from build123d import *

# Parameters (mm, degrees)
BOSS_EXTRUDE1_DEPTH      = 14.5
BOSS_EXTRUDE1_DEPTH_BACK = 14.5
SKETCH2_R                = 1.205
BOSS_EXTRUDE2_DEPTH      = 3.151836
CUT_EXTRUDE1_START       = 9.93575
CUT_EXTRUDE1_DEPTH       = 10
CUT_EXTRUDE2_DEPTH       = 9
CUT_EXTRUDE2_DEPTH_BACK  = 9


with BuildPart() as part:
    # Sketch1 → Boss-Extrude1 (new body, two sides)
    with BuildSketch(Plane.XY) as boss_extrude1_sk:
        with BuildLine():
            Line((5.575, 9.935749893), (13.075, 9.935749893))
            Line((13.075, 9.935749893), (13.075, 3.151836247))
            Line((13.075, 3.151836247), (-13.075, 3.151836247))
            Line((-13.075, 3.151836247), (-13.075, 9.935749893))
            Line((-13.075, 9.935749893), (-5.575, 9.935749893))
            ThreePointArc((-5.575, 9.935749893), (0, 4.360749893), (5.575, 9.935749893))
        make_face()
    extrude(amount=BOSS_EXTRUDE1_DEPTH)
    extrude(boss_extrude1_sk.sketch, amount=-BOSS_EXTRUDE1_DEPTH_BACK)

    # Sketch2 → Boss-Extrude2 (add)
    with BuildSketch(Plane(origin=(0, 0, 0), x_dir=(1, 0, 0), z_dir=(0, 1, 0))):
        with Locations((10.105, 11.46)):
            Circle(SKETCH2_R)
        with Locations((10.026555832, -11.46)):
            Circle(SKETCH2_R)
        with Locations((-10.105, -11.46)):
            Circle(SKETCH2_R)
        with Locations((-10.105, 11.46)):
            Circle(SKETCH2_R)
    extrude(amount=BOSS_EXTRUDE2_DEPTH)

    # Sketch3 → Cut-Extrude1 (cut)
    with BuildSketch(Plane(origin=(0, 0, 0), x_dir=(1, 0, 0), z_dir=(0, 1, 0)).offset(CUT_EXTRUDE1_START)):
        with BuildLine():
            Line((-2.445097234, 3.077415604), (2.391371835, 3.077415604))
            ThreePointArc((2.391371835, 3.077415604), (2.815635904, 2.901679673), (2.991371835, 2.477415604))
            Line((2.991371835, 2.477415604), (2.991371835, -2.51686965))
            ThreePointArc((2.991371835, -2.51686965), (2.815635904, -2.941133719), (2.391371835, -3.11686965))
            Line((2.391371835, -3.11686965), (-2.445097234, -3.11686965))
            ThreePointArc((-2.445097234, -3.11686965), (-2.869361302, -2.941133719), (-3.045097234, -2.51686965))
            Line((-3.045097234, -2.51686965), (-3.045097234, 2.477415604))
            ThreePointArc((-3.045097234, 2.477415604), (-2.869361302, 2.901679673), (-2.445097234, 3.077415604))
        make_face()
    extrude(amount=-CUT_EXTRUDE1_DEPTH, mode=Mode.SUBTRACT)

    # Sketch5 → Cut-Extrude2 (cut, two sides)
    with BuildSketch(Plane.XY) as cut_extrude2_sk:
        with BuildLine():
            Line((-6.450228257, 7.935749893), (-13.075, 7.935749893))
            Line((-13.075, 7.935749893), (-13.075, 3.151836247))
            Line((-13.075, 3.151836247), (13.075, 3.151836247))
            Line((13.075, 3.151836247), (13.075, 7.935749893))
            Line((13.075, 7.935749893), (6.450228257, 7.935749893))
            ThreePointArc((6.450228257, 7.935749893), (0, 3.182569563), (-6.450228257, 7.935749893))
        make_face()
    extrude(amount=CUT_EXTRUDE2_DEPTH, mode=Mode.SUBTRACT)
    extrude(cut_extrude2_sk.sketch, amount=-CUT_EXTRUDE2_DEPTH_BACK, mode=Mode.SUBTRACT)


solid = part.part
Geometry check sheet. Reference: the model listing, model coordinates, mm. A direction names the side the tool comes from. Give positions to 0.01 mm unless a question says otherwise; leave off trailing zeros. Write each loop counter-clockwise with the first axis right and the second up, starting at its lowest first coordinate (ties: lowest second). Pieces come first, ordered by that corner, then holes. Notation, with made-up numbers: M 55,22.5 L 65,22.5 A12 cw 65,36.5 Z; hole C 9.25,84 d5. An arc over 180 degrees is marked long. One line per question, with ' | ' between items.
1. Scan lines: line 1 along Z through (x, y) = (-11.5, 6.25); line 2 along X through (y, z) = (7, 7.5); line 3 along Y through (x, z) = (7, -0.75). Record each from-to range of solid material in increasing order. Write a range as from..to.
Ans:
line 1: -14.5..-9, 9..14.5 | line 2: -6.08..-4.74, 4.74..6.08 | line 3: 7.94..9.94
2. Set-up check for faces 3 (the face through (2.991, 5, 0)), 4 (the face through (11.176, 1.554, 11.098)), 5 (the face through (-13.075, 9, 0)): record each of +Z, -Z, +X, -X, +Y, -Y from which the full face is reachable in a straight line by a thin tool's end or side.
Ans:
face 3: +Y, -Y | face 4: -Y | face 5: +Z, -Z, -X, +Y, -Y
3. Cross-section at A-A (z = -1.25). Enter the section's corners in (x, y) (3 decimals).
Ans:
outline: M -13.075,7.936 L -6.45,7.936 A6.753 ccw -3.045,3.908 L -3.045,5.266 A5.575 cw -5.575,9.936 L -13.075,9.936 Z; M 2.991,3.881 A6.753 ccw 6.45,7.936 L 13.075,7.936 L 13.075,9.936 L 5.575,9.936 A5.575 cw 2.991,5.231 Z
4. Cross-section at C-C (z = -11.46). Enter the section's corners in (x, y) (3 decimals).
Ans:
outline: M -13.075,3.152 L -11.31,3.152 L -11.31,0 L -8.9,0 L -8.9,3.152 L 8.9,3.152 L 8.9,0 L 11.31,0 L 11.31,3.152 L 13.075,3.152 L 13.075,9.936 L 5.575,9.936 A5.575 cw -5.575,9.936 L -13.075,9.936 Z
5. Cross-section at D-D (y = 7). Enter the section's corners in (x, z) (3 decimals), plus the area to 3 significant figures.
Ans:
outline: M -13.075,-14.5 L -4.739,-14.5 L -4.739,14.5 L -13.075,14.5 L -13.075,9 L -6.082,9 L -6.082,-9 L -13.075,-9 Z; M 4.739,-14.5 L 13.075,-14.5 L 13.075,-9 L 6.082,-9 L 6.082,9 L 13.075,9 L 13.075,14.5 L 4.739,14.5 Z | area: 232 mm2
6. Gauge pin test, flat ends, axial feed: pin 1 (4.5 mm diameter, centred on x = 0, z = 10.5, fed in from -Y); pin 2 (3.5 mm diameter, centred on x = -9.5, z = 1.5, fed in from -Y); pin 3 (0.7 mm diameter, centred on y = 4.5, z = -1, fed in from +X). Record the tip position at first contact, or that the pin passes through.
Ans:
pin 1: y = 3.15 | pin 2: y = 7.94 | pin 3: x = 4.44
7. Mould release check, pull along Z, two halves, no side actions. Record for faces 1 (the face through (-10, 0, -11)), 2 (the face through (0, 4, 3.117)): released by +Z, released by -Z, zero draft, split by the parting line, or undercut.
Ans:
face 1: zero draft | face 2: undercut
